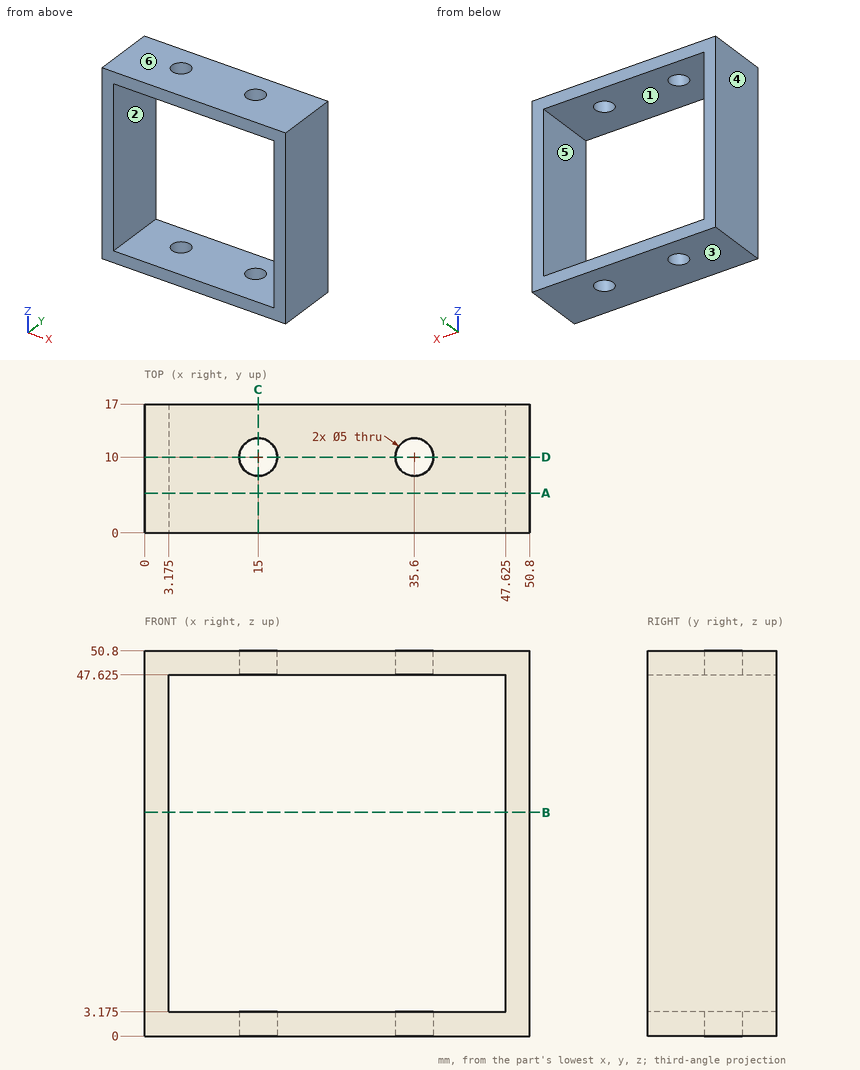
Geometry check sheet. Reference: drawing and pictorial views, mm from the part's lowest x, y, z. A direction names the side the tool comes from. Coordinates: 2 decimals unless noted, no trailing zeros. Order: outer loops, then holes, each group sorted by start corner. A loop starts at its lowest first (then second) coordinate and runs counter-clockwise, first axis right, second up.
Item 1: Section check D-D, the plane y = 10. Enter the section's corners in (x, z) (3 decimals).
Filled in:
outline: (0, 0) - (12.5, 0) - (12.5, 3.175) - (3.175, 3.175) - (3.175, 47.625) - (12.5, 47.625) - (12.5, 50.8) - (0, 50.8) - close; (17.5, 0) - (33.1, 0) - (33.1, 3.175) - (17.5, 3.175) - close; (17.5, 47.625) - (33.1, 47.625) - (33.1, 50.8) - (17.5, 50.8) - close; (38.1, 0) - (50.8, 0) - (50.8, 50.8) - (38.1, 50.8) - (38.1, 47.625) - (47.625, 47.625) - (47.625, 3.175) - (38.1, 3.175) - close
Item 2: Access from +Z, -Z, +X, -X, +Y, -Y to the whole of each face (thin tool, end or side, straight path). Record for the marked faces 5 and 6.
Filled in:
face 5: +Y, -Y
face 6: +Z, +X, -X, +Y, -Y
Item 3: Section check A-A, the plane y = 5.25. Enter the section's corners in (x, z) (3 decimals).
Filled in:
outline: (0, 0) - (50.8, 0) - (50.8, 50.8) - (0, 50.8) - close; hole (3.175, 3.175) - (47.625, 3.175) - (47.625, 47.625) - (3.175, 47.625) - close
Item 4: Release check for a two-part mould opening along X. For the marked faces 1, 2, 3 and 4 record: +X half, -X half, draft (parallel to the pull), parting line (faces both ways), or undercut.
Filled in:
face 1: undercut
face 2: undercut
face 3: draft
face 4: -X half
Item 5: Depth check by flat-ended pin: pin 1 (4.5 mm diameter, centred on x = 35.6, y = 10, fed in from -Z); pin 2 (12 mm diameter, centred on x = 42, z = 38.5, fed in from +Y). Enter the tip coordinate at first touch or a pass-through.
Filled in:
pin 1: passes through
pin 2: stops at y = 17
Item 6: Section check B-B, the plane z = 29.5. Enter the section's corners in (x, y) (3 decimals), then the cut area to 3 significant figures.
Filled in:
outline: (0, 0) - (3.175, 0) - (3.175, 17) - (0, 17) - close; (47.625, 0) - (50.8, 0) - (50.8, 17) - (47.625, 17) - close
area: 108 mm2
Item 7: Section check C-C, the plane x = 15. Enter the section's corners in (y, z) (3 decimals).
Filled in:
outline: (0, 0) - (7.5, 0) - (7.5, 3.175) - (0, 3.175) - close; (0, 47.625) - (7.5, 47.625) - (7.5, 50.8) - (0, 50.8) - close; (12.5, 0) - (17, 0) - (17, 3.175) - (12.5, 3.175) - close; (12.5, 47.625) - (17, 47.625) - (17, 50.8) - (12.5, 50.8) - close
Item 8: Material ranges on L1, parallel to X at y = 10, z = 48.7; L2, parallel to Y at x = 15, z = 49; L3, parallel to Z at x = 43, y = 1 (3 decimals), recorded low to high.
Filled in:
L1: x = 0 to 12.5, 17.5 to 33.1, 38.1 to 50.8
L2: y = 0 to 7.5, 12.5 to 17
L3: z = 0 to 3.175, 47.625 to 50.8
